Build history of the part. All positions in model axes, mm. Face numbers are marked on the shaded views. Round coordinates to 2 decimals unless told otherwise and drop trailing zeros. Order: outer loops, then holes, each group sorted by start corner. A loop starts at its lowest first (then second) coordinate and runs counter-clockwise, first axis right, second up. Notation, with made-up numbers: (-13, -35.75) -> (7, -35.75) arc R16 ccw to (7, -13.75) -> close; hole circle Ø5 at (5, -21). An arc over 180 degrees is marked (long way). Use a Markdown table: item, result. Add a question column.
Item 1: Slice it at D-D, the plane x = -12. Give the cut face in (y, z).
Item 2: Slice it at B-B, the plane x = 0. Give the cut face in (y, z) (3 decimals), plus the area to 3 significant figures.
Item 3: Two-plate mould, pull along X, no slides. Class the marked faces 1, 2 and 3: released by +X, released by -X, zero draft, split by the parting line, or undercut.
Item 4: Slice it at A-A, the plane z = 0. Give the cut face in (x, y) (3 decimals).
Item 5: Pin check, flat tips, straight feed: pin 1 (1.8 mm diameter, centred on y = 13, z = -4.5, fed in from -X); pin 2 (1.8 mm diameter, centred on y = 12, z = -4.5, fed in from +X); pin 3 (2 mm diameter, centred on x = -13.5, y = 5.5, fed in from +Z). Stop position of each tip, or through.
Item 6: Slice it at C-C, the plane y = 4.75. Give the cut face in (x, z) (3 decimals).
Item 7: Probe L1, parallel to Z at x = 0, y = 17.45 (3 decimals); L2, parallel to X at y = 17.35, z = 0 (3 decimals); L3, parallel to Y at x = 3, z = 9. List the from-to ranges inside material, lowest first.
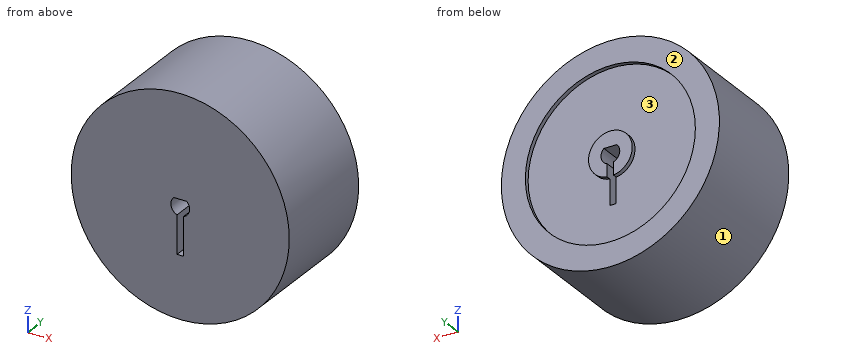
from build123d import *

# Parameters (mm, degrees)
SKETCH1_R           = 17.375
BOSS_EXTRUDE1_DEPTH = 17.7
SKETCH3_R           = 13.545
CUT_EXTRUDE1_DEPTH  = 0.7
SKETCH4_R           = 3.485
BOSS_EXTRUDE2_DEPTH = 0.7
CUT_EXTRUDE2_DEPTH  = 17.7
SKETCH6_W           = 1
SKETCH6_H           = 6.085786438
CUT_EXTRUDE3_DEPTH  = 17.7


with BuildPart() as part:
    # Sketch1 → Boss-Extrude1 (new body)
    with BuildSketch(Plane(origin=(0, 0, 0), x_dir=(1, 0, 0), z_dir=(0, 1, 0))):
        Circle(SKETCH1_R)
    extrude(amount=BOSS_EXTRUDE1_DEPTH)

    # Sketch3 → Cut-Extrude1 (cut)
    with BuildSketch(Plane(origin=(0, 17.7, 0), x_dir=(1, 0, 0), z_dir=(0, 1, 0))):
        Circle(SKETCH3_R)
    extrude(amount=-CUT_EXTRUDE1_DEPTH, mode=Mode.SUBTRACT)

    # Sketch4 → Boss-Extrude2 (add)
    with BuildSketch(Plane(origin=(0, 17, 0), x_dir=(1, 0, 0), z_dir=(0, 1, 0))):
        Circle(SKETCH4_R)
    extrude(amount=BOSS_EXTRUDE2_DEPTH)

    # Sketch5 → Cut-Extrude2 (cut)
    with BuildSketch(Plane(origin=(0, 17.7, 0), x_dir=(1, 0, 0), z_dir=(0, 1, 0))):
        with BuildLine():
            Line((-1.030485323, -1.09), (1.030485323, -1.09))
            ThreePointArc((1.030485323, -1.09), (0, 1.5), (-1.030485323, -1.09))
        make_face()
    extrude(amount=-CUT_EXTRUDE2_DEPTH, mode=Mode.SUBTRACT)

    # Sketch6 → Cut-Extrude3 (cut)
    with BuildSketch(Plane(origin=(0, 17.7, 0), x_dir=(1, 0, 0), z_dir=(0, 1, 0))):
        with Locations((0, 4.457106781)):
            Rectangle(SKETCH6_W, SKETCH6_H)
    extrude(amount=-CUT_EXTRUDE3_DEPTH, mode=Mode.SUBTRACT)


solid = part.part
Check sheet entries:
| question | item | result |
|---|---|---|
| 1 | outline | (0, -12.57) -> (17.7, -12.57) -> (17.7, -6.28) -> (17, -6.28) -> (17, 6.28) -> (17.7, 6.28) -> (17.7, 12.57) -> (0, 12.57) -> close |
| 2 | outline | (0, -17.375) -> (17.7, -17.375) -> (17.7, -13.545) -> (17, -13.545) -> (17, -7.5) -> (0, -7.5) -> close; (0, 1.09) -> (17.7, 1.09) -> (17.7, 3.485) -> (17, 3.485) -> (17, 13.545) -> (17.7, 13.545) -> (17.7, 17.375) -> (0, 17.375) -> close |
| 2 | area | 452 mm2 |
| 3 | face 1 | split by the parting line |
| 3 | face 2 | zero draft |
| 3 | face 3 | undercut |
| 4 | outline | (-17.375, 0) -> (-1.5, 0) -> (-1.5, 17.7) -> (-3.485, 17.7) -> (-3.485, 17) -> (-13.545, 17) -> (-13.545, 17.7) -> (-17.375, 17.7) -> close; (1.5, 0) -> (17.375, 0) -> (17.375, 17.7) -> (13.545, 17.7) -> (13.545, 17) -> (3.485, 17) -> (3.485, 17.7) -> (1.5, 17.7) -> close |
| 5 | pin 1 | x = -17 |
| 5 | pin 2 | x = 17 |
| 5 | pin 3 | z = 12.07 |
| 6 | outline | circle Ø34.75 at (0, 0); hole (-1.03, 1.09) arc R1.5 ccw to (-0.5, -1.414) -> (-0.5, -7.5) -> (0.5, -7.5) -> (0.5, -1.414) arc R1.5 ccw to (1.03, 1.09) -> close |
| 7 | L1 | -17.375 to -13.545, 1.09 to 3.485, 13.545 to 17.375 |
| 7 | L2 | -17.375 to -13.545, -3.485 to -1.5, 1.5 to 3.485, 13.545 to 17.375 |
| 7 | L3 | 0 to 17 |
